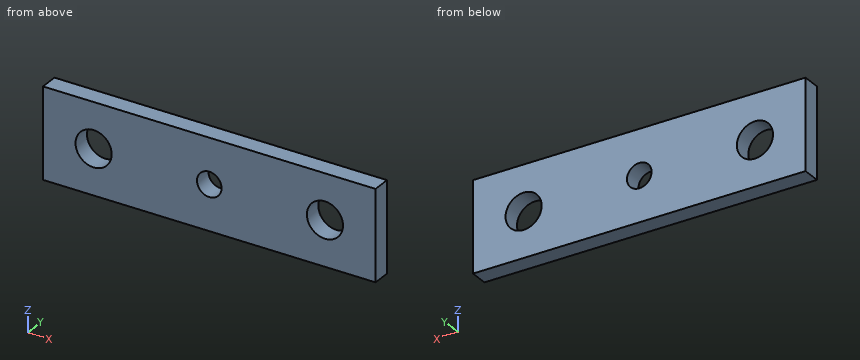
from build123d import *

# Parameters (mm, degrees)
SKETCH_1_W          = 92
SKETCH_1_H          = 25
EXTRUDE_1_DEPTH     = 2.5
SKETCH_2_R          = 5
CUT_EXTRUDE_1_DEPTH = 48.929635926
HOLE_WIZARD_M8_1_D  = 6.8


with BuildPart() as part:
    # 草图1 → 凸台-拉伸1 (new, symmetric)
    with BuildSketch(Plane(origin=(0, 0, 0), x_dir=(1, 0, 0), z_dir=(0, 1, 0))):
        Rectangle(SKETCH_1_W, SKETCH_1_H)
    extrude(amount=EXTRUDE_1_DEPTH, both=True)

    # 草图2 → 切除-拉伸1 (cut, through all)
    with BuildSketch(Plane(origin=(0, 2.5, 0), x_dir=(1, 0, 0), z_dir=(0, 1, 0))):
        with Locations(Location((32, 0, 0), (0, 0, 270))):
            Circle(SKETCH_2_R)
        with Locations(Location((-32, 0, 0), (0, 0, 270))):
            Circle(SKETCH_2_R)
    extrude(amount=-CUT_EXTRUDE_1_DEPTH, mode=Mode.SUBTRACT)

    # M8 螺纹孔1 (through all)
    with Locations(Plane(origin=(0, 2.5, 0), x_dir=(1, 0, 0), z_dir=(0, 1, 0))):
        with Locations((0, 0)):
            Hole(HOLE_WIZARD_M8_1_D / 2)


solid = part.part
Verification items for the finished model (mm, model axes). Give positions to 0.01 mm unless a question says otherwise; leave off trailing zeros. Write each loop counter-clockwise with the first axis right and the second up, starting at its lowest first coordinate (ties: lowest second). Pieces come first, ordered by that corner, then holes.
(1) Cross-section at B-B (z = 0). Enter the section's corners in (x, y).
(2) Material ranges on line 1 (X direction, y = 1.5, z = 4.5); line 2 (Z direction, x = 0, y = -1.5); line 3 (Z direction, x = -30.5, y = -1.6), recorded low to high.
(3) Cross-section at D-D (x = 32). Enter the section's corners in (y, z).
(4) Cross-section at C-C (y = -1.2). Enter the section's corners in (x, z), plus the area to 3 significant figures.
(5) Cross-section at A-A (x = 0). Enter the section's corners in (y, z), plus the area to 3 significant figures.
Worked out:
1. outline: (-46, -2.5) - (-37, -2.5) - (-37, 2.5) - (-46, 2.5) - close; (-27, -2.5) - (-3.4, -2.5) - (-3.4, 2.5) - (-27, 2.5) - close; (3.4, -2.5) - (27, -2.5) - (27, 2.5) - (3.4, 2.5) - close; (37, -2.5) - (46, -2.5) - (46, 2.5) - (37, 2.5) - close
2. line 1: x = -46 to -34.18, -29.82 to 29.82, 34.18 to 46
2. line 2: z = -12.5 to -3.4, 3.4 to 12.5
2. line 3: z = -12.5 to -4.77, 4.77 to 12.5
3. outline: (-2.5, -12.5) - (2.5, -12.5) - (2.5, -5) - (-2.5, -5) - close; (-2.5, 5) - (2.5, 5) - (2.5, 12.5) - (-2.5, 12.5) - close
4. outline: (-46, -12.5) - (46, -12.5) - (46, 12.5) - (-46, 12.5) - close; hole circle Ø10 at (-32, 0); hole circle Ø6.8 at (0, 0); hole circle Ø10 at (32, 0)
4. area: 2,110 mm2
5. outline: (-2.5, -12.5) - (2.5, -12.5) - (2.5, -3.4) - (-2.5, -3.4) - close; (-2.5, 3.4) - (2.5, 3.4) - (2.5, 12.5) - (-2.5, 12.5) - close
5. area: 91.0 mm2
